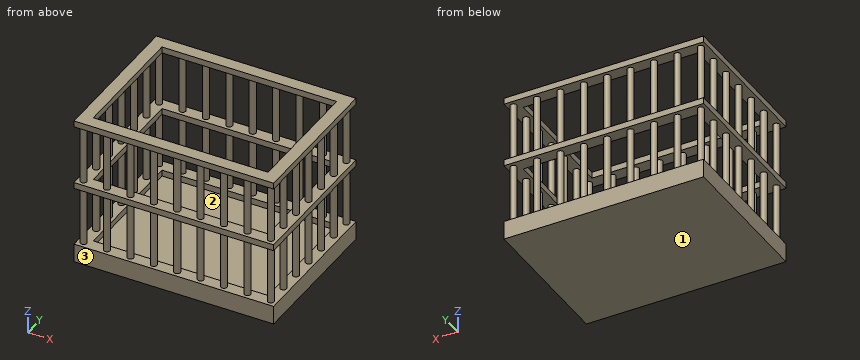
from build123d import *

# Parameters (mm, degrees)
F0_W     = 101.6
F0_H     = 76.2
F0_W_2   = 88.9
F0_H_2   = 63.5
F1_DEPTH = 1.5875
F2_R     = 1.5875
F3_DEPTH = 31.75
F4_W     = 101.6
F4_H     = 76.2
F4_W_2   = 88.9
F4_H_2   = 63.5
F5_DEPTH = 3.175
F6_W     = 101.6
F6_H     = 76.2
F6_W_2   = 88.9
F6_H_2   = 63.5
F7_DEPTH = 3.175
F8_W     = 101.6
F8_H     = 76.2
F9_DEPTH = 6.35


with BuildPart() as f1:
    # F0 (on Top) → F1 (new body, symmetric)
    with BuildSketch(Plane.XY):
        with Locations((-50.8, 38.1)):
            Rectangle(F0_W, F0_H)
        with Locations((-50.8, 38.1)):
            Rectangle(F0_W_2, F0_H_2, mode=Mode.SUBTRACT)
    extrude(amount=F1_DEPTH, both=True)

    # F2 (on Top) → F3 (join, symmetric)
    with BuildSketch(Plane.XY):
        with Locations((-98.425, 3.175)):
            Circle(F2_R)
        with Locations((-86.51875, 3.175)):
            Circle(F2_R)
        with Locations((-74.6125, 3.175)):
            Circle(F2_R)
        with Locations((-38.89375, 73.025)):
            Circle(F2_R)
        with Locations((-98.425, 26.458333)):
            Circle(F2_R)
        with Locations((-98.425, 14.816667)):
            Circle(F2_R)
        with Locations((-62.70625, 73.025)):
            Circle(F2_R)
        with Locations((-3.175, 49.741667)):
            Circle(F2_R)
        with Locations((-3.175, 61.383333)):
            Circle(F2_R)
        with Locations((-3.175, 73.025)):
            Circle(F2_R)
        with Locations((-15.08125, 73.025)):
            Circle(F2_R)
        with Locations((-50.8, 3.175)):
            Circle(F2_R)
        with Locations((-62.70625, 3.175)):
            Circle(F2_R)
        with Locations((-26.9875, 73.025)):
            Circle(F2_R)
        with Locations((-3.175, 14.816667)):
            Circle(F2_R)
        with Locations((-3.175, 26.458333)):
            Circle(F2_R)
        with Locations((-3.175, 38.1)):
            Circle(F2_R)
        with Locations((-3.175, 3.175)):
            Circle(F2_R)
        with Locations((-15.08125, 3.175)):
            Circle(F2_R)
        with Locations((-26.9875, 3.175)):
            Circle(F2_R)
        with Locations((-38.89375, 3.175)):
            Circle(F2_R)
        with Locations((-98.425, 49.741667)):
            Circle(F2_R)
        with Locations((-74.6125, 73.025)):
            Circle(F2_R)
        with Locations((-98.425, 38.1)):
            Circle(F2_R)
        with Locations((-50.8, 73.025)):
            Circle(F2_R)
        with Locations((-98.425, 73.025)):
            Circle(F2_R)
        with Locations((-86.51875, 73.025)):
            Circle(F2_R)
        with Locations((-98.425, 61.383333)):
            Circle(F2_R)
    extrude(amount=F3_DEPTH, both=True)

    # F4 (on face) → F5 (join)
    with BuildSketch(Plane.XY.offset(31.75)):
        with Locations((-50.8, 38.1)):
            Rectangle(F4_W, F4_H)
        with Locations((-50.8, 38.1)):
            Rectangle(F4_W_2, F4_H_2, mode=Mode.SUBTRACT)
    extrude(amount=F5_DEPTH)

    # F6 (on face) → F7 (join)
    with BuildSketch(Plane(origin=(0, 0, -31.75), x_dir=(1, 0, 0), z_dir=(0, 0, -1))):
        with Locations((-50.8, -38.1)):
            Rectangle(F6_W, F6_H)
        with Locations((-50.8, -38.1)):
            Rectangle(F6_W_2, F6_H_2, mode=Mode.SUBTRACT)
    extrude(amount=F7_DEPTH)

    # F8 (on face) → F9 (join)
    with BuildSketch(Plane(origin=(0, 0, -34.925), x_dir=(1, 0, 0), z_dir=(0, 0, -1))):
        with Locations((-50.8, -38.1)):
            Rectangle(F8_W, F8_H)
    extrude(amount=F9_DEPTH)


solid = f1.part
Design review of the part built by this model. Coordinates are the model's own, in mm. Face numbers are marked on the shaded views. Round coordinates to 2 decimals unless told otherwise and drop trailing zeros.
1) Consider section A-A (x = -24). Count the separate pieces of the cut face and the enclosed holes in it, plus the area to 3 significant figures.
The answers:
separate pieces: 5
enclosed holes: 0
area: 605 mm2
2) Clearance check with flat-ended pins moving along their axes: pin 1 Ø10 at (x, y) = (-21, 14) entering from +Z (3 decimals); pin 2 Ø4 at (x, z) = (-37, 23.5) entering from +Y; pin 3 Ø4 at (y, z) = (17.5, 24) entering from +X. State where each tip first meets the part, or that it passes through.
The answers:
pin 1: stops at z = -34.925
pin 2: stops at y = 74.61
pin 3: stops at x = -1.74
3) Draft analysis for pull direction Z (two halves, no side actions). For the marked faces 1, 2 and 3, state which applies: released by +Z, released by -Z, zero draft, split by the parting line, or undercut.
The answers:
face 1: released by -Z
face 2: released by +Z
face 3: zero draft
4) For L1, parallel to Y at x = -74.5, z = -3; L2, parallel to Y at x = -50.5, z = 24; L3, parallel to Z at x = -85, y = 54 (3 decimals), list the stretches that pass through material, from the lowest coordinate up.
The answers:
L1: y = 1.59 to 4.76, 71.44 to 74.61
L2: y = 1.62 to 4.73, 71.47 to 74.58
L3: z = -41.275 to -34.925
